For this review, take the finished solid that the model builds, in its own axes (mm). A direction names the side the tool comes from. Coordinates: 2 decimals unless noted, no trailing zeros. Order: outer loops, then holes, each group sorted by start corner. A loop starts at its lowest first (then second) coordinate and runs counter-clockwise, first axis right, second up. Notation, with made-up numbers: (24, 50) -> (71, 50) arc R9 ccw to (71, 66) -> close; hole circle Ø1 at (-9, -35). An arc over 180 degrees is marked (long way). Return JSON: item names as keys, results as strings. Group by question number.
Item 1: Take a section at B-B (x = -13.5). Write out the cut boundary in (y, z), then the cut area to 3 significant figures.
Item 2: Draft analysis for pull direction X (two halves, no side actions). For faces 6 (the flat face through (-44.196, -5, 9)), 7 (the flat face through (-32, 0, 0)), 8 (the cylindrical face through (-53.588, 7.559, -5.796)), state which applies: +X half, -X half, draft (parallel to the pull), parting line (faces both ways), or undercut.
Item 3: Take a section at C-C (z = -15). Write out the cut boundary in (x, y).
Item 4: Take a section at A-A (y = 0). Write out the cut boundary in (x, z) (3 decimals).
Item 5: Machinability: for faces 1 (the cylindrical face through (6.26, -15.12, -11.59)), 2 (the flat face through (29.21, 11, -4)), 3 (the cylindrical face through (-29.094, 0.813, 6.44)), 4 (the flat face through (0, 4, -12.4)), 5 (the conical face through (66.865, -2.373, -10.687)), which of the approach directions +Z, -Z, +X, -X, +Y, -Y give a long, thin tool a straight path to every point of the face, cutting with its end or side? Answer none if there is none.
Item 6: For line 1 along X through (y, z) = (0, 5); line 2 along X through (y, z) = (6.5, -11.5); line 3 along X through (y, z) = (-1.5, 0.5), list the stretches that pass through material, from the lowest coordinate up.
Item 7: Insertion check: pin 1 (6 mm diameter, centred on x = -31.67, y = 0, fed in from -Z); pin 2 (5 mm diameter, centred on x = -44.5, y = -3.5, fed in from +Z); pin 3 (1.5 mm diameter, centred on x = 37, z = 13, fed in from +Y); pin 4 (5 mm diameter, centred on x = -46, z = -12, fed in from -Y). Each pin has a flat end and moves straight along its axis. Give the tip position at first contact, or say it passes through.
```python
from build123d import *

# Parameters (mm, degrees)
F0_R      = 19.05
F1_DEPTH  = 12.7
F2_R      = 12.7
F3_DEPTH  = 44.196
F4_R      = 9.525
F5_DEPTH  = 19.05
F6_R      = 11.3538
F7_DEPTH  = 16.51
F8_R      = 11.8872
F8_R_2    = 11.3538
F9_DEPTH  = 74.2696
F9_TAPER  = 1.43
F11_R     = 2.7051
F12_DEPTH = 12.7


with BuildPart() as f1:
    # F0 (on Right) → F1 (new body)
    with BuildSketch(Plane.YZ):
        Circle(F0_R)
    extrude(amount=F1_DEPTH)

    # F2 (on face) → F3 (join)
    with BuildSketch(Plane(origin=(0, 0, 0), x_dir=(0, -1, 0), z_dir=(-1, 0, 0))):
        Circle(F2_R)
    extrude(amount=F3_DEPTH)

    # F4 (on face) → F5 (join)
    with BuildSketch(Plane(origin=(-44.196, 0, 0), x_dir=(0, -1, 0), z_dir=(-1, 0, 0))):
        Circle(F4_R)
    extrude(amount=F5_DEPTH)

    # F6 (on face) → F7 (join)
    with BuildSketch(Plane.YZ.offset(12.7)):
        Circle(F6_R)
    extrude(amount=F7_DEPTH)

    # F8 (on face) → F9 (join)
    with BuildSketch(Plane.YZ.offset(29.21)):
        Circle(F8_R)
        Circle(F8_R_2, mode=Mode.SUBTRACT)
        Circle(F8_R_2)
    extrude(amount=F9_DEPTH, taper=F9_TAPER)

    # F11 (on offset) → F12 (cut)
    with BuildSketch(Plane.XY.offset(12.7)):
        with Locations((-31.6738, 0)):
            Circle(F11_R)
    extrude(amount=-F12_DEPTH, mode=Mode.SUBTRACT)


solid = f1.part
```
Findings below:
{
 "1": {"outline": "circle Ø25.4 at (0, 0)", "area": "507 mm2"},
 "2": {"face 6": "-X half", "face 7": "undercut", "face 8": "draft"},
 "3": {"outline": "(0, -11.74) -> (12.7, -11.74) -> (12.7, 11.74) -> (0, 11.74) -> close"},
 "4": {"outline": "(-63.246, -9.525) -> (-44.196, -9.525) -> (-44.196, -12.7) -> (0, -12.7) -> (0, -19.05) -> (12.7, -19.05) -> (12.7, -11.354) -> (29.21, -11.354) -> (29.21, -11.887) -> (103.48, -10.033) -> (103.48, 10.033) -> (29.21, 11.887) -> (29.21, 11.354) -> (12.7, 11.354) -> (12.7, 19.05) -> (0, 19.05) -> (0, 12.7) -> (-28.969, 12.7) -> (-28.969, 0) -> (-34.379, 0) -> (-34.379, 12.7) -> (-44.196, 12.7) -> (-44.196, 9.525) -> (-63.246, 9.525) -> close"},
 "5": {"face 1": "+X, -X", "face 2": "none", "face 3": "+Z", "face 4": "-X", "face 5": "+X"},
 "6": {"line 1": "x = -63.25 to -34.38, -28.97 to 103.48", "line 2": "x = 0 to 12.7", "line 3": "x = -63.25 to -33.92, -29.42 to 103.48"},
 "7": {"pin 1": "stops at z = -12.7", "pin 2": "stops at z = 12.66", "pin 3": "passes through", "pin 4": "stops at y = -7.47"}
}
